Work out the finished part from the listing and answer in its coordinate system (mm). A direction names the side the tool comes from. Round coordinates to 2 decimals unless told otherwise and drop trailing zeros. Write each loop counter-clockwise with the first axis right and the second up, starting at its lowest first coordinate (ties: lowest second). Pieces come first, ordered by that corner, then holes. Notation, with made-up numbers: (20.25, 75.5) -> (61.25, 75.5) arc R24 cw to (61.25, 98.5) -> close; hole circle Ø10 at (17.25, 7.5). An arc over 180 degrees is marked (long way). One line per item, written item: value.
Autodesk Inventor part; units mm, degrees
ref_plane "YZ Plane" through (0, 0, 0) normal (1, 0, 0) x (0, 1, 0)
ref_plane "XZ Plane" through (0, 0, 0) normal (0, 1, 0) x (-1, 0, 0)
ref_plane "XY Plane" through (0, 0, 0) normal (0, 0, 1) x (1, 0, 0)
sketch "Sketch1" plane through (0, 0, 0) normal (0, 0, 1) x (1, 0, 0)
  line L0 (0, 0) -> (240, 0)
  line L1 (240, 0) -> (240, 240)
  line L2 (240, 240) -> (0, 240)
  line L3 (0, 240) -> (0, 0)
  dimension "d0" = 240
  dimension "d1" = 240
extrude "Extrusion1" add sketch "Sketch1" along normal blind 240
sketch "Sketch2" plane through (0, 0, 240) normal (0, 0, 1) x (1, 0, 0)
  line L0 (30, 210) -> (210, 210)
  line L1 (210, 210) -> (210, 30)
  line L2 (210, 30) -> (30, 30)
  line L3 (30, 30) -> (30, 210)
  line L4 (240, 240) -> (0, 240)
  line L5 (0, 240) -> (0, 0)
  line L6 (240, 0) -> (240, 240)
  line L7 (0, 0) -> (240, 0)
  dimension "d4" = 30
  dimension "d5" = 30
  dimension "d6" = 30
  dimension "d7" = 30
extrude "Extrusion2" cut sketch "Sketch2" against normal blind 500 contours L0 L1 L2 L3
sketch "Sketch3" plane through (0, 240, 0) normal (0, 1, 0) x (1, 0, 0)
  line L0 (30, -30) -> (210, -30)
  line L1 (210, -30) -> (210, -210)
  line L2 (210, -210) -> (30, -210)
  line L3 (30, -210) -> (30, -30)
  line L4 (240, 0) -> (0, 0)
  line L5 (0, 0) -> (0, -240)
  line L6 (240, 0) -> (240, -240)
  line L7 (240, -240) -> (0, -240)
  dimension "d10" = 30
  dimension "d11" = 30
  dimension "d12" = 30
  dimension "d13" = 30
extrude "Extrusion3" cut sketch "Sketch3" against normal blind 500 contours L0 L1 L2 L3
sketch "Sketch4" plane through (240, 0, 0) normal (1, 0, 0) x (0, 0, -1)
  line L0 (-240, 210) -> (-210, 210)
  line L1 (-30, 30) -> (-30, 0)
  line L2 (-210, 210) -> (-30, 210)
  line L3 (-30, 210) -> (-30, 30)
  line L4 (-30, 30) -> (-210, 30)
  line L5 (-210, 30) -> (-210, 210)
  point P0 (0, 0)
extrude "Extrusion4" cut sketch "Sketch4" against normal blind 500
sketch "Sketch5" plane through (0, 0, 240) normal (0, 0, 1) x (1, 0, 0)
  line L0 (0, 0) -> (240, 0)
  line L1 (240, 240) -> (0, 240)
  line L2 (0, 0) -> (10, 0)
  line L3 (10, 0) -> (10, 240)
  line L4 (10, 240) -> (0, 240)
  line L5 (0, 240) -> (0, 0)
  line L6 (10, 240) -> (240, 240)
  line L7 (240, 240) -> (240, 230)
  line L8 (240, 230) -> (10, 230)
  line L9 (10, 230) -> (10, 240)
  line L10 (10, 0) -> (240, 0)
  line L11 (240, 0) -> (240, 10)
  line L12 (240, 10) -> (10, 10)
  line L13 (10, 10) -> (10, 0)
  line L14 (240, 230) -> (230, 230)
  line L15 (230, 230) -> (230, 10)
  line L16 (230, 10) -> (240, 10)
  line L17 (240, 10) -> (240, 230)
  dimension "d18" = 10
  dimension "d19" = 10
  dimension "d20" = 10
  dimension "d21" = 10
extrude "Extrusion5" cut sketch "Sketch5" against normal blind 900 contours L5 L1 L3 L0 | L3 L12 L11 L0 | L1 L7 L8 L3 | L12 L15 L8 L17
sketch "Sketch6" plane through (10, 230, 240) normal (0, 1, 0) x (1, 0, 0)
  line L0 (0, 240) -> (220.3242, 240)
  line L1 (220.3242, 240) -> (220.3242, 230)
  line L2 (220.3242, 230) -> (0, 230)
  line L3 (0, 230) -> (0, 240)
  line L4 (0, 0) -> (220, 0)
  line L5 (220, 0) -> (220, 240)
  line L6 (0, 0) -> (220, 0)
  line L7 (220, 0) -> (220, 10)
  line L8 (220, 10) -> (0, 10)
  line L9 (0, 10) -> (0, 0)
  point P0 (-10, 240)
  dimension "d24" = 10
  dimension "d25" = 10
extrude "Extrusion6" cut sketch "Sketch6" against normal blind 900
sketch "Sketch10" plane through (10, 230, 230) normal (0, 1, 0) x (1, 0, 0)
  line L0 (0, 0) -> (0, 220)
  line L1 (220, 20) -> (200, 20)
  line L2 (0, 0) -> (220, 0)
  line L3 (220, 0) -> (220, 20)
  line L4 (220, 20) -> (0, 20)
  line L5 (0, 20) -> (0, 0)
  point P0 (-10, 230)
extrude "Extrusion7" cut sketch "Sketch10" against normal blind 900
sketch "Sketch11" plane through (230, 30, 30) normal (1, 0, 0) x (0, 0, -1)
  line L0 (-180, 0) -> (0, 0)
  line L1 (0, 180) -> (-180, 180)
  line L2 (-180, 0) -> (-160, 0)
  line L3 (-160, 0) -> (-160, 180)
  line L4 (-160, 180) -> (-180, 180)
  line L5 (-180, 180) -> (-180, 0)
  point P0 (30, -30)
  dimension "d31" = 20
extrude "Extrusion8" add sketch "Sketch11" against normal blind 220
sketch "Sketch12" plane through (30, 210, 210) normal (0, 1, 0) x (1, 0, 0)
  line L0 (180, 180) -> (180, 20)
  line L1 (0, 0) -> (180, 0)
  line L2 (180, 0) -> (180, 20)
  line L3 (180, 20) -> (0, 20)
  line L4 (0, 20) -> (0, 0)
  point P0 (-30, 210)
extrude "Extrusion9" add sketch "Sketch12" along normal blind 20
sketch "Sketch13" plane through (30, 30, 190) normal (0, -1, 0) x (1, 0, 0)
  line L0 (0, 0) -> (-20, 0)
  line L1 (180, 20) -> (0, 20)
  line L2 (0, 20) -> (0, 0)
  line L3 (0, 0) -> (180, 0)
  line L4 (180, 0) -> (180, 20)
  point P0 (-30, -190)
extrude "Extrusion10" add sketch "Sketch13" along normal blind 20
sketch "Sketch14" plane through (10, 230, 210) normal (0, 0, 1) x (1, 0, 0)
  line L0 (220, -20) -> (200, -20)
  line L1 (20, -200) -> (20, -20)
  line L2 (200, -20) -> (20, -20)
  line L3 (20, -20) -> (20, -200)
  line L4 (20, -200) -> (200, -200)
  line L5 (200, -200) -> (200, -20)
  point P0 (-10, -230)
extrude "Extrusion11" cut sketch "Sketch14" against normal blind 20
properties part number "Gearbox Housing"
(1) Find section C-C on z = 195. Give the vertices of the cut face in (x, y), plus the area to 3 significant figures.
Reported:
outline: (10, 10) -> (230, 10) -> (230, 230) -> (10, 230) -> close; hole (30, 30) -> (210, 30) -> (210, 210) -> (30, 210) -> close
area: 16,000 mm2
(2) For a pull along Z with two mould halves and no side action, classify faces 1 (the face through (119, 220, 30)), 2 (the face through (121, 210, 200)), 3 (the face through (24, 122, 10)) as pulls with the +Z half, pulls with the -Z half, needs draft (parallel to the pull), parting line crosses it, or undercut.
Reported:
face 1: undercut
face 2: needs draft
face 3: pulls with the -Z half
(3) A tool of negligible diameter and unlimited length cuts with its end or side. For faces 4 (the face through (118, 10, 23)), 5 (the face through (30, 220, 111)), 6 (the face through (119, 30, 200)), 7 (the face through (10, 122, 23)), 8 (the face through (220, 210, 111)), from which of +Z, -Z, +X, -X, +Y, -Y can it reach the whole face along a straight path? Write none if from no direction.
Reported:
face 4: +Z, -Z, +X, -X, -Y
face 5: +Y, -Y
face 6: +Z, -Z
face 7: +Z, -Z, -X, +Y, -Y
face 8: +X, -X
(4) Find section B-B on z = 166.5. Give the vertices of the cut face in (x, y).
Reported:
outline: (10, 10) -> (30, 10) -> (30, 30) -> (10, 30) -> close; (10, 210) -> (30, 210) -> (30, 230) -> (10, 230) -> close; (210, 10) -> (230, 10) -> (230, 30) -> (210, 30) -> close; (210, 210) -> (230, 210) -> (230, 230) -> (210, 230) -> close
(5) Consider probe 1 along Y at (x, z) = (99, 29.5). Determine where the line is inside the solid, lowest interval first.
Reported:
probe 1: y = 10 to 30, 210 to 230
(6) Find section A-A on y = 154. Give the vertices of the cut face in (x, z).
Reported:
outline: (10, 10) -> (30, 10) -> (30, 30) -> (10, 30) -> close; (10, 190) -> (30, 190) -> (30, 210) -> (10, 210) -> close; (210, 10) -> (230, 10) -> (230, 30) -> (210, 30) -> close; (210, 190) -> (230, 190) -> (230, 210) -> (210, 210) -> close
